Source: CAD feature listing. Evaluate the final solid. Frame: model axes, mm. A direction names the side the tool comes from. Give positions to 0.01 mm unless a question says otherwise; leave off trailing zeros. Order: outer loops, then holes, each group sorted by start corner. A loop starts at its lowest first (then second) coordinate and runs counter-clockwise, first axis right, second up. Notation, with made-up numbers: M 71.25,75 L 93.25,75 A9 ccw 93.25,84 Z; hole C -38,-2 d8. An arc over 180 degrees is marked long. Return JSON: item names as keys, results as strings.
from build123d import *

# Parameters (mm, degrees)
F0_R     = 8
F1_DEPTH = 7.8
F0_R_2   = 15
F2_DEPTH = 3.5
F3_DEPTH = 7.8
F4_COUNT = 12
F6_DEPTH = 3.5
F8_R     = 0.25
F9_COUNT = 30


with BuildPart() as f1:
    # F0 (on Front) → F1 (new body)
    with BuildSketch(Plane.XZ):
        Circle(F0_R)
        with BuildLine():
            ThreePointArc((0.25, 6.229985955), (4.4963304483, 4.3195182023), (6.235, 0))
            ThreePointArc((6.235, 0), (-4.3195182023, -4.4963304483), (-0.25, 6.229985955))
            ThreePointArc((-0.25, 6.229985955), (0, 6.235), (0.25, 6.229985955))
        make_face(mode=Mode.SUBTRACT)
    extrude(amount=F1_DEPTH)

    # F0 (on Front) → F2 (join)
    with BuildSketch(Plane.XZ):
        Circle(F0_R_2)
        Circle(F0_R, mode=Mode.SUBTRACT)
    extrude(amount=F2_DEPTH)

    # F4: F3 ×12 about axis
    f4_axis = Axis((0, 0, 0), (0, -1, 0))


with BuildPart() as f3:
    # F0 (on Front) → F3 (new body)
    with BuildSketch(Plane.XZ):
        with BuildLine():
            Line((0.25, 5.993085955), (0.25, 6.229985955))
            ThreePointArc((0.25, 6.229985955), (0, 6.235), (-0.25, 6.229985955))
            Line((-0.25, 6.229985955), (-0.25, 5.993085955))
            Line((-0.25, 5.993085955), (0.25, 5.993085955))
        make_face()
    extrude(amount=F3_DEPTH)


with BuildPart() as f1_1:
    add(f1.part)
    for i in range(1, F4_COUNT):
        add(f3.part.rotate(f4_axis, i * 360 / F4_COUNT))



with BuildPart() as f6:
    # F5 (on Front) → F6 (new body)
    with BuildSketch(Plane.XZ):
        with BuildLine():
            Line((1.894147114, 16.894147114), (0, 15))
            ThreePointArc((0, 15), (1.6713062771, 14.9066003947), (3.321799308, 14.6275647104))
            Line((3.321799308, 14.6275647104), (1.894147114, 16.894147114))
        make_face()
    extrude(amount=F6_DEPTH)

    # F8
    f8_edges = [f6.edges().sort_by_distance(p)[0] for p in [
        (1.894147, -1.75, 16.894147),
    ]]
    fillet(f8_edges, radius=F8_R)


with BuildPart() as f1_2:
    add(f1_1.part)

    add(f3.part)  # F9 merges F3

    add(f6.part)  # F9 merges F6
    # F9: F6 ×30 about axis
    f9_axis = Axis((0, -8.9512197301, 0), (0, -1, 0))
    for i in range(1, F9_COUNT):
        add(f6.part.rotate(f9_axis, i * 360 / F9_COUNT))


solid = f1_2.part
1. Ray query, probe 1 along Z at (x, y) = (-14.5, -1.5); probe 2 along Y at (x, z) = (-10.5, 3.5); probe 3 along X at (y, z) = (-3, 0.5). Return the intervals inside material, ascending.
Evaluation:
{"probe 1": "z = -7.1 to -4.76, -4.52 to 4.69, 5.09 to 7.27", "probe 2": "y = -3.5 to 0", "probe 3": "x = -16.51 to -6.21, 6.21 to 16.24"}
2. Set-up query: faces 1 (the face through (-5.645, -1.726, 14.891)), 2 (the face through (-14.91, -1.73, -5.54)), 3 (the face through (2.426, -1.726, -15.739)). Return all of +Z, -Z, +X, -X, +Y, -Y with unobstructed straight access to the full face (end or side cutting, diameter ignored); none if empty.
Evaluation:
{"face 1": "+Z, +Y, -Y", "face 2": "-X, +Y, -Y", "face 3": "-Z, +Y, -Y"}
3. Section query A-A (z = 1). Return loops of the section in (x, y), then the cut area to 3 significant figures.
Evaluation:
{"outline": "M -15.88,-3.5 L -7.94,-3.5 L -7.94,-7.8 L -6.15,-7.8 L -6.15,0 L -15.88,0 Z; M 6.15,-7.8 L 7.94,-7.8 L 7.94,-3.5 L 15.62,-3.5 L 15.62,0 L 6.15,0 Z", "area": "82.5 mm^2"}
4. Section query C-C (z = -11). Return loops of the section in (x, y), then the cut area to 4 significant figures.
Evaluation:
{"outline": "M -11.36,-3.5 L 11.2,-3.5 L 11.2,0 L -11.36,0 Z", "area": "78.95 mm^2"}
5. First-contact query: pin 1 (2 mm diameter, centred on x = 9, z = 7, fed in from -Y). Flat tip, straight axial feed; report the tip coordinate or a pass-through.
Evaluation:
{"pin 1": "stops at y = -3.5"}
6. Section query B-B (x = -7.5). Return loops of the section in (y, z).
Evaluation:
{"outline": "M -7.8,-2.78 L -3.5,-2.78 L -3.5,-14.24 L 0,-14.24 L 0,14.42 L -3.5,14.42 L -3.5,2.78 L -7.8,2.78 Z"}
7. Draft query along Z for faces 4 (the face through (8.62, -1.73, -13.39)), 5 (the face through (15.73, -1.73, 2.31)), 6 (the face through (-3.947, -1.726, 15.404)). Return one class per face: pulls with the +Z half, pulls with the -Z half, needs draft (parallel to the pull), parting line crosses it, or undercut.
Evaluation:
{"face 4": "pulls with the -Z half", "face 5": "undercut", "face 6": "pulls with the +Z half"}
